from build123d import *

# Parameters (mm, degrees)
F0_W      = 134.552986
F0_H      = 74.75166
F1_DEPTH  = 30
F3_DEPTH  = 8
F4_W      = 125.513256
F4_H      = 63.625834
F5_DEPTH  = 20
F6_W      = 16.467378
F6_H      = 14.950332
F7_DEPTH  = 2
F8_W      = 3.476821
F8_H      = 15.298014
F9_DEPTH  = 10
F10_W     = 21.382451
F10_H     = 15.298014
F11_DEPTH = 5
F12_R     = 5


with BuildPart() as f1:
    # F0 (on Top) → F1 (new body)
    with BuildSketch(Plane.XY):
        Rectangle(F0_W, F0_H)
    extrude(amount=F1_DEPTH)

    # F2 (on face) → F3 (cut)
    with BuildSketch(Plane.XY.offset(30)):
        with BuildLine():
            Line((8.233689, -24.47048), (8.233689, 24.47048))
            Line((8.233689, 24.47048), (-3.233689, 24.47048))
            ThreePointArc((-3.233689, 24.47048), (-6.769223, 23.006014), (-8.233689, 19.47048))
            Line((-8.233689, 19.47048), (-8.233689, -19.47048))
            ThreePointArc((-8.233689, -19.47048), (-6.769223, -23.006014), (-3.233689, -24.47048))
            Line((-3.233689, -24.47048), (8.233689, -24.47048))
        make_face()
    extrude(amount=-F3_DEPTH, mode=Mode.SUBTRACT)

    # F4 (on face) → F5 (cut)
    with BuildSketch(Plane(origin=(0, 0, 0), x_dir=(1, 0, 0), z_dir=(0, 0, -1))):
        Rectangle(F4_W, F4_H)
    extrude(amount=-F5_DEPTH, mode=Mode.SUBTRACT)

    # F6 (on face) → F7 (cut, through all)
    with BuildSketch(Plane.XY.offset(22)):
        Rectangle(F6_W, F6_H)
    extrude(amount=-F7_DEPTH, mode=Mode.SUBTRACT)

    # F8 (on face) → F9 (join)
    with BuildSketch(Plane(origin=(0, 0, 20), x_dir=(1, 0, 0), z_dir=(0, 0, -1))):
        with Locations((-31.291391, 0)):
            Rectangle(F8_W, F8_H)
        with Locations((31.291391, 0)):
            Rectangle(F8_W, F8_H)
    extrude(amount=F9_DEPTH)

    # F10 (on face) → F11 (join)
    with BuildSketch(Plane(origin=(0, 0, 10), x_dir=(1, 0, 0), z_dir=(0, 0, -1))):
        with Locations((-40.244206, 0)):
            Rectangle(F10_W, F10_H)
        with Locations((40.244206, 0)):
            Rectangle(F10_W, F10_H)
    extrude(amount=F11_DEPTH)

    # F12
    f12_edges = [f1.edges().sort_by_distance(p)[0] for p in [
        (-50.935432, -7.649007, 7.5),
        (-50.935432, 7.649007, 7.5),
        (50.935432, 7.649007, 7.5),
        (50.935432, -7.649007, 7.5),
    ]]
    fillet(f12_edges, radius=F12_R)


solid = f1.part
Check sheet for the modelled part. Datum: model origin and axes. Units: mm. A direction names the side the tool comes from. Give positions to 0.01 mm unless a question says otherwise; leave off trailing zeros. Loops run counter-clockwise (first coordinate to the right, second up) from the corner with the lowest first, then second, coordinate; pieces in that order, holes last. Notation, with made-up numbers: M 27,1 L 66,1 A27 cw 66,21 Z; hole C 65.5,9.25 d8. An arc over 180 degrees is marked long. Return JSON: item names as keys, results as strings. Group by question number.
1. Cross-section at B-B on z = 8.25. Record the boundary of the cut face in (x, y).
2. Cross-section at D-D on y = 15. Record the boundary of the cut face in (x, z).
3. Tool access check on faces 4 (the flat face through (42, 0, 10)), 5 (the cylindrical face through (49.51, -6.145, 7.465)), 6 (the flat face through (0, -16, 22)), 7 (the flat face through (-1, 37.376, 15)). Record the directions out of +Z, -Z, +X, -X, +Y, -Y that give a thin tool (end or side, any length) a straight path to the whole face; none if there is none.
4. Cross-section at A-A on x = -1.5. Record the boundary of the cut face in (y, z).
5. Cross-section at C-C on y = 4.5. Record the boundary of the cut face in (x, z), plus the area to 3 significant figures.
6. Thickness scan on L1, parallel to X at y = -1.5, z = 11.5; L2, parallel to Y at x = -55, z = 3.25; L3, parallel to X at y = -4.5, z = 7. Record the ranges inside material, lowest first.
7. Mould release check, pull along Y, two halves, no side actions. Record for faces 1 (the flat face through (3, 24.47, 26)), 2 (the flat face through (-16, 1, 30)), 3 (the flat face through (-1, -37.376, 15)): released by +Y, released by -Y, zero draft, split by the parting line, or undercut.
8. Go/stop test with flat-tipped pins: pin 1 (8 mm diameter, centred on x = -11.5, y = 24.5, fed in from -Z); pin 2 (7.5 mm diameter, centred on x = 42, y = 1, fed in from -Z). Record where each tip stops, or that it passes through.
Return value:
{
 "1": {"outline": "M -67.28,-37.38 L 67.28,-37.38 L 67.28,37.38 L -67.28,37.38 Z; M -50.94,-2.65 A5 ccw -45.94,-7.65 L -29.55,-7.65 L -29.55,7.65 L -45.94,7.65 A5 ccw -50.94,2.65 Z; M 29.55,-7.65 L 45.94,-7.65 A5 ccw 50.94,-2.65 L 50.94,2.65 A5 ccw 45.94,7.65 L 29.55,7.65 Z; hole M -62.76,-31.81 L 62.76,-31.81 L 62.76,31.81 L -62.76,31.81 Z"},
 "2": {"outline": "M -67.28,0 L -62.76,0 L -62.76,20 L 62.76,20 L 62.76,0 L 67.28,0 L 67.28,30 L 8.23,30 L 8.23,22 L -8.23,22 L -8.23,30 L -67.28,30 Z"},
 "3": {"face 4": "none", "face 5": "-Z", "face 6": "+Z", "face 7": "+Z, -Z, +X, -X, +Y"},
 "4": {"outline": "M -37.38,0 L -31.81,0 L -31.81,20 L -7.48,20 L -7.48,22 L -24.47,22 L -24.47,30 L -37.38,30 Z; M 7.48,20 L 31.81,20 L 31.81,0 L 37.38,0 L 37.38,30 L 24.47,30 L 24.47,22 L 7.48,22 Z"},
 "5": {"outline": "M -67.28,0 L -62.76,0 L -62.76,20 L -33.03,20 L -33.03,10 L -50.58,10 L -50.58,5 L -29.55,5 L -29.55,20 L -8.23,20 L -8.23,30 L -67.28,30 Z; M 8.23,20 L 29.55,20 L 29.55,5 L 50.58,5 L 50.58,10 L 33.03,10 L 33.03,20 L 62.76,20 L 62.76,0 L 67.28,0 L 67.28,30 L 8.23,30 Z", "area": "1,640 mm^2"},
 "6": {"L1": "-67.28 to -62.76, -33.03 to -29.55, 29.55 to 33.03, 62.76 to 67.28", "L2": "-37.38 to -31.81, 31.81 to 37.38", "L3": "-67.28 to -62.76, -50.58 to -29.55, 29.55 to 50.58, 62.76 to 67.28"},
 "7": {"face 1": "undercut", "face 2": "zero draft", "face 3": "released by -Y"},
 "8": {"pin 1": "z = 20", "pin 2": "z = 5"}
}
